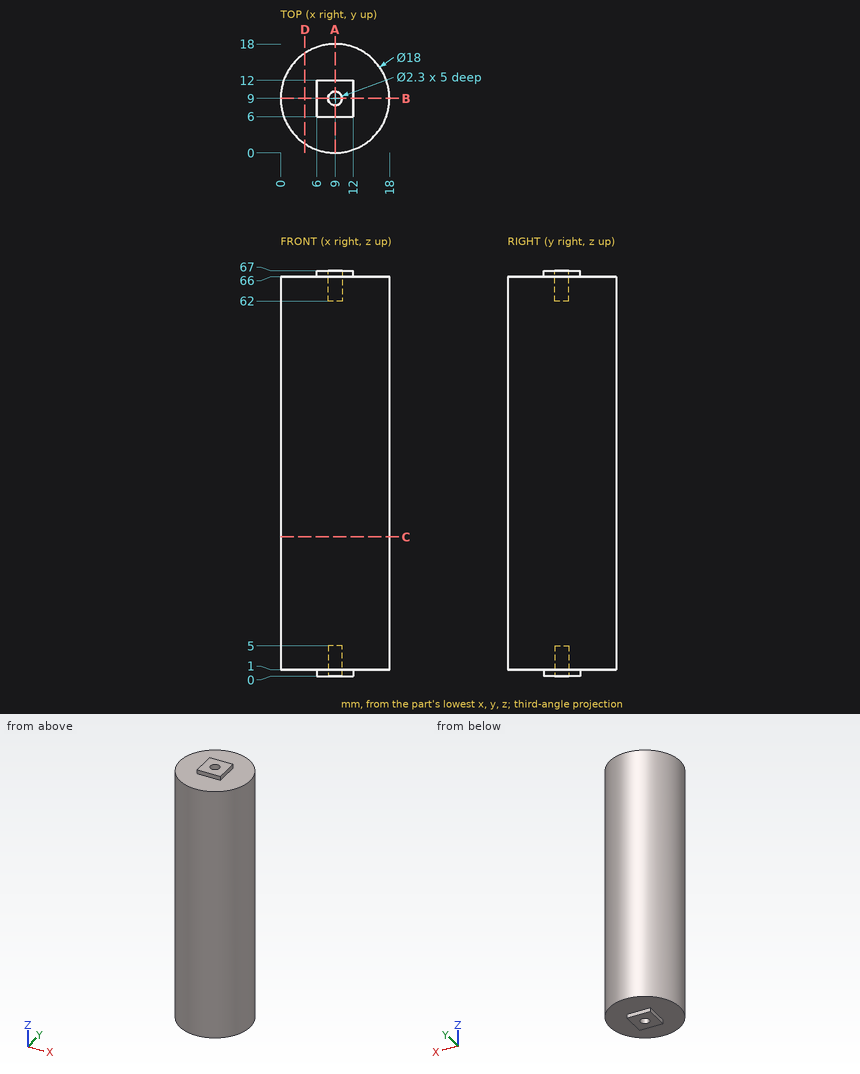
Geometry check sheet. Reference: drawing and pictorial views, mm from the part's lowest x, y, z. Round coordinates to 2 decimals unless told otherwise and drop trailing zeros. Write each loop counter-clockwise with the first axis right and the second up, starting at its lowest first coordinate (ties: lowest second). Pieces come first, ordered by that corner, then holes.
1. Scan lines: L1, parallel to Y at x = 9, z = 65; L2, parallel to Z at x = 9, y = 15.25; L3, parallel to Y at x = 4, z = 23.5. Record each from-to range of solid material in increasing order.
2. Section check D-D on x = 4. Enter the section's corners in (y, z), plus the area to 3 significant figures.
3. Section check C-C on z = 23. Enter the section's corners in (x, y).
4. Gauge pin test, flat ends, axial feed: P1, Ø0.5, axis at x = 7.5, z = 0.5, coming from the +Y side; P2, Ø0.5, axis at y = 7.5, z = 66.5, coming from the +X side; P3, Ø5, axis at x = 2, y = 13, coming from the -Z side. Record the tip position at first contact, or that the pin passes through.
5. Section check A-A on x = 9. Enter the section's corners in (y, z), plus the area to 3 significant figures.
Answer:
1. L1: y = 0 to 7.85, 10.15 to 18
1. L2: z = 1 to 66
1. L3: y = 1.52 to 16.48
2. outline: (1.52, 1) - (16.48, 1) - (16.48, 66) - (1.52, 66) - close
2. area: 973 mm2
3. outline: circle Ø18 at (9, 9)
4. P1: stops at y = 12
4. P2: stops at x = 12
4. P3: stops at z = 1
5. outline: (0, 1) - (6, 1) - (6, 0) - (7.85, 0) - (7.85, 5) - (10.15, 5) - (10.15, 0) - (12, 0) - (12, 1) - (18, 1) - (18, 66) - (12, 66) - (12, 67) - (10.15, 67) - (10.15, 62) - (7.85, 62) - (7.85, 67) - (6, 67) - (6, 66) - (0, 66) - close
5. area: 1,160 mm2
